Can you work these out from the drawing? Everything is in mm from the part's minimum corner. Round coordinates to 2 decimals unless told otherwise and drop trailing zeros. Loops run counter-clockwise (first coordinate to the right, second up) from the corner with the lowest first, then second, coordinate; pieces in that order, holes last. Notation, with made-up numbers: (53.5, -8) - (82.5, -8) arc R19 ccw to (82.5, 23) - close; hole circle Ø4 at (55.25, 57). An arc over 180 degrees is marked (long way). Answer as a JSON object with one key per item and string values. Group by question number.
1) I want a section at A-A, the plane y = 25. Please give me the cut outline in (x, z).
2) I want a section at B-B, the plane z = 14.5. Please give me the cut outline in (x, y).
3) I want a section at C-C, the plane x = 1.4. Please give me the cut outline in (y, z).
4) If I drill on line 1 along Z through (x, y) = (1.2, 25); line 2 along Z through (x, y) = (0.6, 24); line 3 along Y through (x, z) = (0.35, 18.5), over which ranges is the centre line in solid material (lowest first)? Write a range as [from, to].
5) I want a section at D-D, the plane y = 35.5. Please give me the cut outline in (x, z).
6) Will these pins go through, and if not, where does the flat tip stop? P1, Ø1, axis at x = 1, z = 19, coming from the +Y side; P2, Ø0.6, axis at x = 0.5, z = 19, coming from the -Y side (1 decimal); P3, Ø1, axis at x = 1, y = 20, coming from the -Z side; P4, Ø3, axis at y = 25, z = 14.5, coming from the +X side.
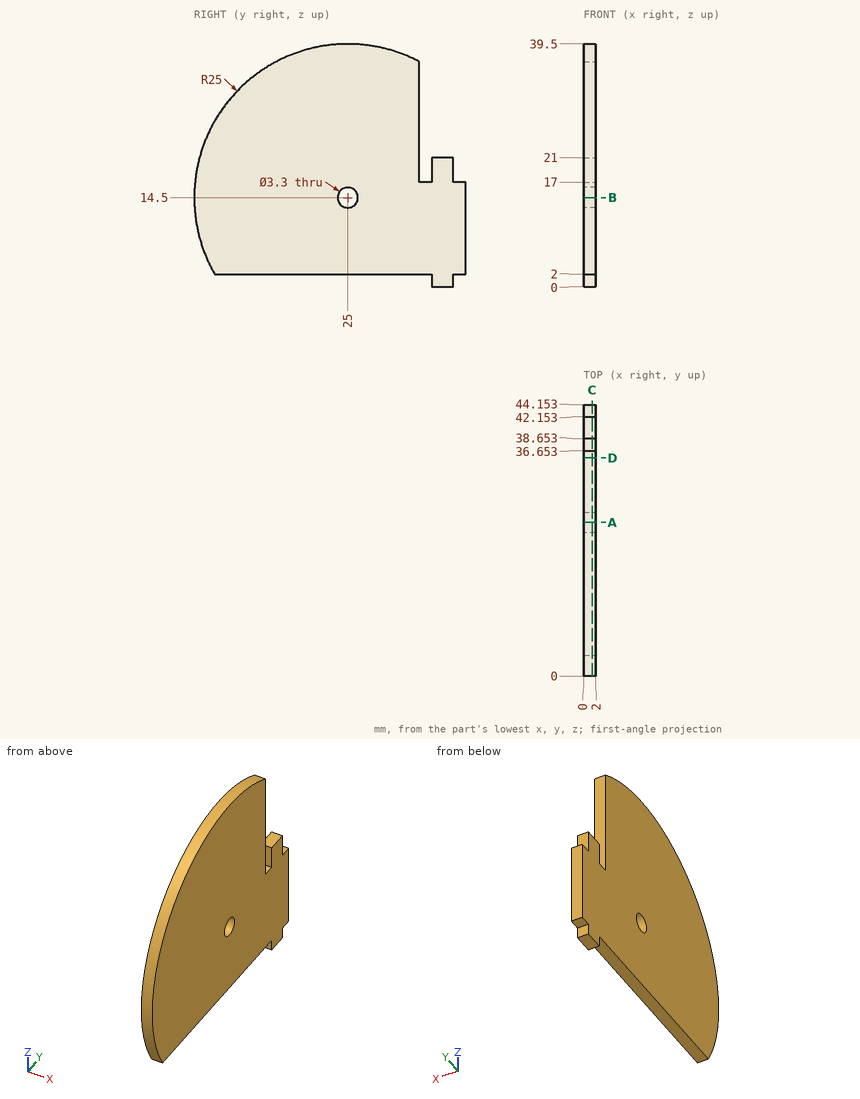
Outcome:
{
 "1": {"outline": "(0, 2) - (2, 2) - (2, 12.85) - (0, 12.85) - close; (0, 16.15) - (2, 16.15) - (2, 39.5) - (0, 39.5) - close"},
 "2": {"outline": "(0, 0) - (2, 0) - (2, 23.35) - (0, 23.35) - close; (0, 26.65) - (2, 26.65) - (2, 44.15) - (0, 44.15) - close"},
 "3": {"outline": "(3.35, 2) - (38.65, 2) - (38.65, 0) - (42.15, 0) - (42.15, 2) - (44.15, 2) - (44.15, 17) - (42.15, 17) - (42.15, 21) - (38.65, 21) - (38.65, 17) - (36.65, 17) - (36.65, 36.62) arc R25 ccw to start; hole circle Ø3.3 at (25, 14.5)"},
 "4": {"line 1": "[2, 12.85], [16.15, 39.5]", "line 2": "[2, 13.19], [15.81, 39.48]", "line 3": "[0.32, 36.65], [38.65, 42.15]"},
 "5": {"outline": "(0, 2) - (2, 2) - (2, 37.19) - (0, 37.19) - close"},
 "6": {"P1": "y = 42.15", "P2": "y = 0.4", "P3": "z = 2", "P4": "through"}
}
